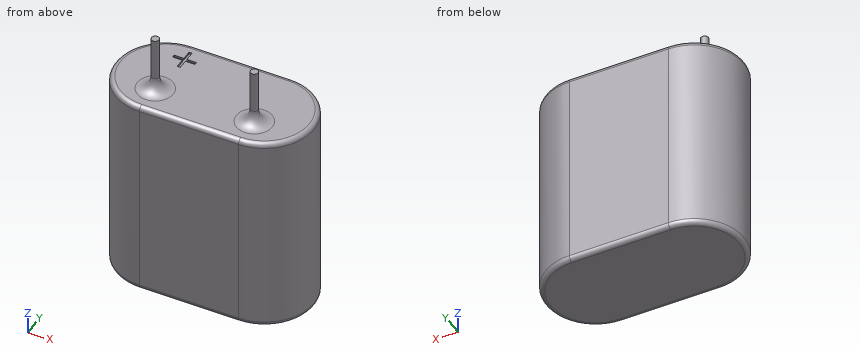
from build123d import *

# Parameters (mm, degrees)
BOSS_EXTRUDE1_DEPTH = 22
SKETCH2_R           = 0.4
FILLET1_R           = 1.5
FILLET2_R           = 0.5
CUT_EXTRUDE1_DEPTH  = 0.2


with BuildPart() as part:
    # Sketch1 → Boss-Extrude1 (new body)
    with BuildSketch(Plane.XY):
        with BuildLine():
            Line((0, 5.25), (10.5, 5.25))
            ThreePointArc((10.5, 5.25), (15.75, 0), (10.5, -5.25))
            Line((10.5, -5.25), (0, -5.25))
            ThreePointArc((0, -5.25), (-5.25, 0), (0, 5.25))
        make_face()
    extrude(amount=-BOSS_EXTRUDE1_DEPTH)

    # Sweep1: sweep along a path in Sketch3
    with BuildLine(Plane.YZ) as sweep1_path:
        Line((-2.05, 0), (-2.05, 6))
    # Sketch2 → Sweep1 (sweep)
    with BuildSketch(Plane.XY):
        with Locations((0, -2.05)):
            Circle(SKETCH2_R)
        with Locations((10.5, -2.05)):
            Circle(SKETCH2_R)
    sweep(path=sweep1_path.line)

    # Fillet1
    fillet1_edges = [part.edges().sort_by_distance(p)[0] for p in [
        (-0.4, -2.05, 0),
        (10.1, -2.05, 0),
    ]]
    fillet(fillet1_edges, radius=FILLET1_R)

    # Fillet2
    fillet2_edges = [part.edges().sort_by_distance(p)[0] for p in [
        (15.75, 0, -22),
        (5.25, 5.25, -22),
        (-5.25, 0, -22),
        (5.25, 5.25, 0),
        (15.75, 0, 0),
        (5.25, -5.25, 0),
        (-5.25, 0, 0),
        (5.25, -5.25, -22),
    ]]
    fillet(fillet2_edges, radius=FILLET2_R)

    # Sketch4 → Cut-Extrude1 (cut)
    with BuildSketch(Plane.XY):
        Polygon((0.301282051, 3.134615385), (0.301282051, 4.166666667), (0.615384615, 4.166666667), (0.615384615, 3.134615385), (1.647435897, 3.134615385), (1.647435897, 2.820512821), (0.615384615, 2.820512821), (0.615384615, 1.788461538), (0.301282051, 1.788461538), (0.301282051, 2.820512821), (-0.730769231, 2.820512821), (-0.730769231, 3.134615385), align=None)
    extrude(amount=-CUT_EXTRUDE1_DEPTH, mode=Mode.SUBTRACT)


solid = part.part
Geometry: final body of the model. Coordinates: model frame, mm. Coordinates: 2 decimals unless noted, no trailing zeros. Loops run counter-clockwise (first coordinate to the right, second up) from the corner with the lowest first, then second, coordinate; pieces in that order, holes last. Notation, with made-up numbers: M 42.25,-34.75 L 73.25,-34.75 A14 cw 73.25,-26.75 Z; hole C 2,87.25 d2. An arc over 180 degrees is marked long. One line per item, written item: value. Start each with the question number.
1) Cut plane A-A (x = 3.5). Return loops of the section in (y, z).
2) Cut plane B-B (z = 3). Return loops of the section in (x, y), then the cut area to 3 significant figures.
3) Pin query (flat end, axial travel): P1, Ø4, axis at y = 3, z = -12, coming from the +X side; P2, Ø5, axis at x = 7, y = 2, coming from the +Z side; P3, Ø1.5, axis at y = 1.5, z = -4, coming from the -X side. Return the tip coordinate at first contact, or that it passes through.
4) Material intervals for L1, parallel to Z at x = 1.5, y = 2.75; L2, parallel to X at y = -0.25, z = -1.5; L3, parallel to X at y = -2.25, z = -14.75, sorted ascending. Write a range as from..to.
5) Cut plane C-C (z = -9). Return loops of the section in (x, y), then the cut area to 3 significant figures.
Evaluation:
1. outline: M -5.25,-21.5 A0.5 ccw -4.75,-22 L 4.75,-22 A0.5 ccw 5.25,-21.5 L 5.25,-0.5 A0.5 ccw 4.75,0 L -4.75,0 A0.5 ccw -5.25,-0.5 Z
2. outline: C 0,-2.05 d0.8; C 10.5,-2.05 d0.8
2. area: 1.01 mm^2
3. P1: x = 15.65
3. P2: z = 0
3. P3: x = -5.2
4. L1: -22..0
4. L2: -5.24..15.74
4. L3: -4.74..15.24
5. outline: M 0,-5.25 L 10.5,-5.25 A5.25 ccw 10.5,5.25 L 0,5.25 A5.25 ccw Z
5. area: 197 mm^2
